Here's how the part is built. I have some questions about the finished solid (model axes, mm). A direction names the side the tool comes from. Round coordinates to 2 decimals unless told otherwise and drop trailing zeros. Loops run counter-clockwise (first coordinate to the right, second up) from the corner with the lowest first, then second, coordinate; pieces in that order, holes last. Notation, with made-up numbers: M -18.5,32 L 10.5,32 A30 ccw 10.5,70 Z; hole C -15.75,-6.5 d5. An arc over 180 degrees is marked long. Write item = value, one per line. Start each with the question number.
from build123d import *

# Parameters (mm, degrees)
F0_W      = 25
F0_H      = 20
F0_W_2    = 15
F0_H_2    = 30
F1_DEPTH  = 25
F2_R      = 5.25
F3_DEPTH  = 65.001
F4_R      = 2
F5_DEPTH  = 25
F6_R      = 3
F7_R      = 2
F8_DEPTH  = 65.001
F9_R      = 3.25
F10_DEPTH = 55.001


with BuildPart() as f1:
    # F0 (on Front) → F1 (new body)
    with BuildSketch(Plane.XZ):
        Polygon((12.5, 10), (12.5, -10), (-12.5, -10), (12.5, -25), (27.5, -25), align=None)
        Rectangle(F0_W, F0_H)
        with Locations((20, -40)):
            Rectangle(F0_W_2, F0_H_2)
    extrude(amount=F1_DEPTH)

    # F2 (on face) → F3 (cut, through all)
    with BuildSketch(Plane.XY.offset(10)):
        with Locations((0, -12.5)):
            Circle(F2_R)
    extrude(amount=-F3_DEPTH, mode=Mode.SUBTRACT)

    # F4 (on face) → F5 (cut)
    with BuildSketch(Plane(origin=(12.5, 0, 0), x_dir=(0, -1, 0), z_dir=(-1, 0, 0))):
        with Locations((19.25, -30.1)):
            Circle(F4_R)
        with Locations((5.75, -49.9)):
            Circle(F4_R)
        with Locations((5.75, -30.1)):
            Circle(F4_R)
        with Locations((19.25, -49.9)):
            Circle(F4_R)
    extrude(amount=-F5_DEPTH, mode=Mode.SUBTRACT)

    # F6
    f6_edges = [f1.edges().sort_by_distance(p)[0] for p in [
        (-12.5, -25, 0),
        (-12.5, 0, 0),
        (-12.5, -12.5, -10),
        (0, -25, -17.5),
        (0, 0, -17.5),
        (12.5, -12.5, -25),
        (12.5, -12.5, -55),
        (20, -25, -7.5),
        (20, 0, -7.5),
        (20, -25, -55),
        (20, 0, -55),
        (12.5, 0, -40),
        (12.5, -25, -40),
    ]]
    fillet(f6_edges, radius=F6_R)

    # F7 (on face) → F8 (cut, through all)
    with BuildSketch(Plane.XY.offset(10)):
        with Locations((-5.6568542495, -6.8431457505)):
            Circle(F7_R)
        with Locations((5.6568542495, -18.1568542495)):
            Circle(F7_R)
    extrude(amount=-F8_DEPTH, mode=Mode.SUBTRACT)

    # F9 (on Top) → F10 (cut, through all)
    with BuildSketch(Plane.XY):
        with Locations((-5.6611075997, -6.9247833453)):
            Circle(F9_R)
        with Locations((5.6935697794, -18.1814264506)):
            Circle(F9_R)
    extrude(amount=-F10_DEPTH, mode=Mode.SUBTRACT)


solid = f1.part
Item 1: Please list where these lines run through material, in increasing order: line 1 (Y direction, x = 0, z = -13); line 2 (Y direction, x = 19, z = -31); line 3 (Z direction, x = -4, y = -5.25). Write a range as [from, to].
Item 2: For faces 4 (the flat face through (12.5, -12, -40)), 5 (the cylindrical face through (19.895, -18.816, -32.052)), 6 (the cylindrical face through (13.4, -0.86, -39.17)), 7 (the cylindrical face through (-6.182, -3.717, -6.131)), which set-ups out of +Z, -Z, +X, -X, +Y, -Y let a thin tool reach every point of the face, with its end or its side?
Item 3: I want a section at D-D, the plane y = -5.75. List the corners of the cut face in (x, z) for me.
Item 4: I want a section at A-A, the plane z = -49.9. List the corners of the cut face in (x, y) for me.
Item 5: I want a section at B-B, the plane y = -12.5. List the corners of the cut face in (x, z) for me.
Item 6: I want a section at C-C, the plane y = -19.25. List the corners of the cut face in (x, z) for me.
Item 7: We'd pull the mould along Y, two halves only. Please class faces 1 (the cylindrical face through (20.17, -0.86, -10.18)), 2 (the flat face through (7, -20, 0)), 3 (the flat face through (20.105, -12.367, -7.745)): released by +Y, released by -Y, zero draft, split by the parting line, or undercut.
Item 8: Will these pins go through, and if not, where does the flat tip stop? pin 1 Ø7.5 at (x, y) = (-5.66, -6.92) entering from -Z; pin 2 Ø6.5 at (y, z) = (-19.25, -30.1) entering from -X; pin 3 Ø2.5 at (x, y) = (-5.66, -6.84) entering from -Z; pin 4 Ø7 at (x, y) = (6, -16.5) entering from -Z.
Worked out:
q1.line_1 = [-25, -17.75], [-7.25, 0]
q1.line_2 = [-25, -21.04], [-17.46, -7.54], [-3.96, 0]
q1.line_3 = [0, 10]
q2.face_4 = -Z, -X, +Y, -Y
q2.face_5 = +X, -X
q2.face_6 = -Z, -X, +Y
q2.face_7 = -Z
q3.outline = M -12.5,-8.3 A3 ccw -11.04,-10.87 L -8.69,-12.29 L -8.69,0 L -7.33,0 L -7.33,10 L -12.5,10 Z; M -3.98,0 L -2.63,0 L -2.63,-15.92 L 11.04,-24.13 A3 cw 12.5,-26.7 L 12.5,-28.1 L 27.5,-28.1 L 27.5,-25 L 12.5,10 L -3.98,10 Z; M 12.5,-52 A3 ccw 15.5,-55 L 27.5,-55 L 27.5,-51.9 L 12.5,-51.9 Z; M 12.5,-47.9 L 27.5,-47.9 L 27.5,-32.1 L 12.5,-32.1 Z
q4.outline = M 12.5,-22 A3 ccw 15.5,-25 L 27.5,-25 L 27.5,-21.25 L 12.5,-21.25 Z; M 12.5,-17.25 L 27.5,-17.25 L 27.5,-7.75 L 12.5,-7.75 Z; M 12.5,-3.75 L 27.5,-3.75 L 27.5,0 L 15.5,0 A3 ccw 12.5,-3 Z
q5.outline = M -12.5,-8.3 A3 ccw -11.04,-10.87 L -5.25,-14.35 L -5.25,10 L -12.5,10 Z; M 5.25,-20.65 L 11.04,-24.13 A3 cw 12.5,-26.7 L 12.5,-52 A3 ccw 15.5,-55 L 27.5,-55 L 27.5,-25 L 12.5,10 L 5.25,10 Z
q6.outline = M -12.5,-8.3 A3 ccw -11.04,-10.87 L 2.62,-19.07 L 2.62,0 L 3.98,0 L 3.98,10 L -12.5,10 Z; M 7.33,0 L 8.76,0 L 8.76,-22.76 L 11.04,-24.13 A3 cw 12.5,-26.7 L 12.5,-28.1 L 27.5,-28.1 L 27.5,-25 L 12.5,10 L 7.33,10 Z; M 12.5,-52 A3 ccw 15.5,-55 L 27.5,-55 L 27.5,-51.9 L 12.5,-51.9 Z; M 12.5,-47.9 L 27.5,-47.9 L 27.5,-32.1 L 12.5,-32.1 Z
q7.face_1 = released by +Y
q7.face_2 = undercut
q7.face_3 = zero draft
q8.pin_1 = -16.35
q8.pin_2 = 12.5
q8.pin_3 = through
q8.pin_4 = -23.2
